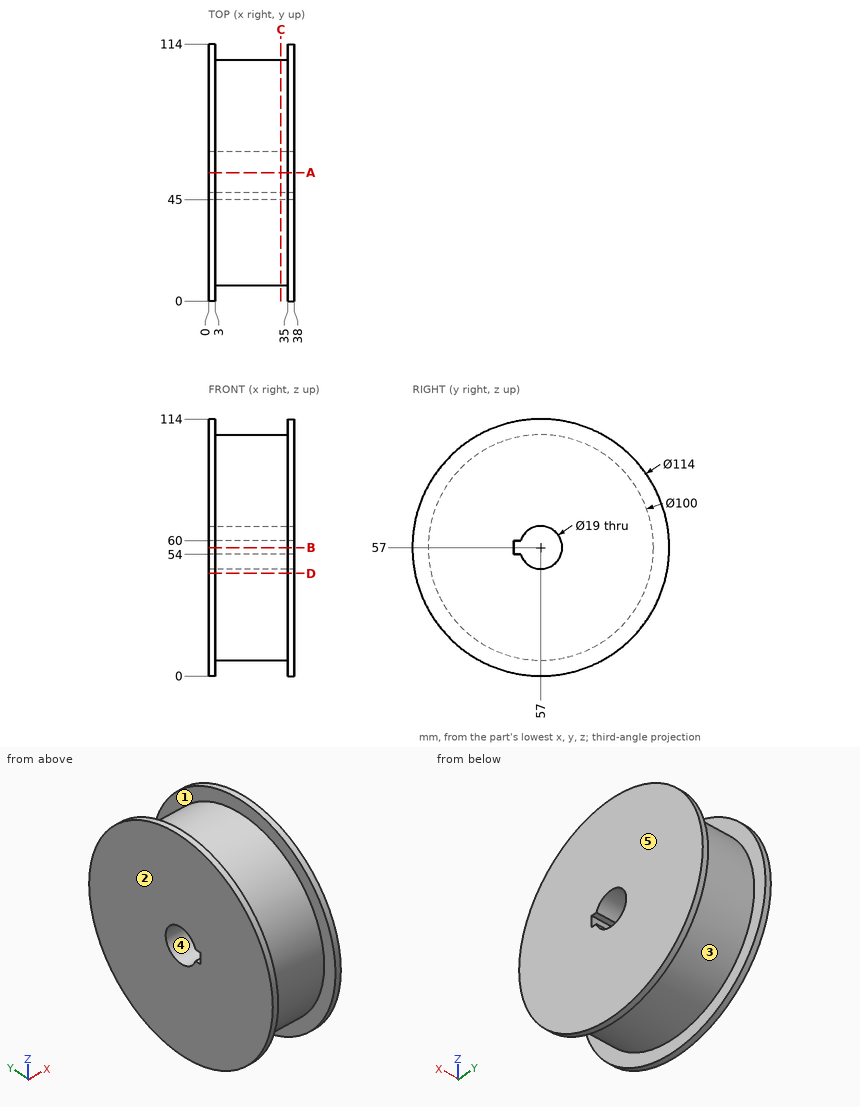
Source: three-view drawing plus pictorial views. Frame: mm from the lowest corner of the part. A direction names the side the tool comes from. Give positions to 0.01 mm unless a question says otherwise; leave off trailing zeros. Order: outer loops, then holes, each group sorted by start corner. A loop starts at its lowest first (then second) coordinate and runs counter-clockwise, first axis right, second up. Notation, with made-up numbers: M 80,68 L 123,68 A28 cw 123,100 Z; hole C 35.5,-25 d2. An arc over 180 degrees is marked long. Return JSON: item names as keys, results as strings.
Item 1: Cut plane D-D (z = 45.5). Return loops of the section in (x, y), then the cut area to 3 significant figures.
Solutions:
{"outline": "M 0,1.17 L 3,1.17 L 3,8.34 L 35,8.34 L 35,1.17 L 38,1.17 L 38,112.83 L 35,112.83 L 35,105.66 L 3,105.66 L 3,112.83 L 0,112.83 Z", "area": "3,780 mm^2"}
Item 2: Pull-direction query (X, two-part tool) for the marked faces 3, 4 and 5; classes: +X half, -X half, draft (parallel to the pull), parting line (faces both ways), or undercut.
Solutions:
{"face 3": "undercut", "face 4": "draft", "face 5": "+X half"}
Item 3: Cut plane A-A (y = 57). Return loops of the section in (x, z), then the cut area to 3 significant figures.
Solutions:
{"outline": "M 0,0 L 3,0 L 3,7 L 35,7 L 35,0 L 38,0 L 38,47.5 L 0,47.5 Z; M 0,66.5 L 38,66.5 L 38,114 L 35,114 L 35,107 L 3,107 L 3,114 L 0,114 Z", "area": "3,160 mm^2"}
Item 4: Cut plane B-B (z = 57). Return loops of the section in (x, y), then the cut area to 3 significant figures.
Solutions:
{"outline": "M 0,0 L 3,0 L 3,7 L 35,7 L 35,0 L 38,0 L 38,45 L 0,45 Z; M 0,66.5 L 38,66.5 L 38,114 L 35,114 L 35,107 L 3,107 L 3,114 L 0,114 Z", "area": "3,070 mm^2"}
Item 5: First-contact query: P1, Ø1, axis at x = 11.5, y = 19.5, coming from the +Z side; P2, Ø2, axis at x = 18, z = 31, coming from the -Y side; P3, Ø0.9, axis at x = 20.5, y = 46, coming from the -Z side. Flat tips, straight axial feed; report the tip coordinate or a pass-through.
Solutions:
{"P1": "z = 90.63", "P2": "y = 13.7", "P3": "z = 8.13"}
Item 6: Access query for the marked faces 1 and 2. Directions: +Z, -Z, +X, -X, +Y, -Y. A direction counts if a zero-diameter tool reaches every point of the face in a straight line with its end or side. Return the directions, or none.
Solutions:
{"face 1": "none", "face 2": "+Z, -Z, -X, +Y, -Y"}
Item 7: Cut plane C-C (x = 32). Return loops of the section in (y, z), then the cut area to 3 significant figures.
Solutions:
{"outline": "C 57,57 d100; hole M 45,54 L 47.99,54 A9.5 ccw long 47.99,60 L 45,60 Z", "area": "7,550 mm^2"}
Item 8: Ray query, probe 1 along X at (y, z) = (31, 104.5); probe 2 along Z at (x, y) = (25.5, 57); probe 3 along Y at (x, z) = (13, 57.5). Return the intervals inside material, ascending.
Solutions:
{"probe 1": "0 to 3, 35 to 38", "probe 2": "7 to 47.5, 66.5 to 107", "probe 3": "7 to 45, 66.49 to 107"}
